```python
from build123d import *

# Parameters (mm, degrees)
SKETCH28_W          = 12.7
SKETCH28_H          = 12.7
BOSS_EXTRUDE5_DEPTH = 9.525
SKETCH29_W          = 12.7
SKETCH29_H          = 12.7
BOSS_EXTRUDE6_DEPTH = 9.525
SKETCH30_R          = 2.286
CUT_EXTRUDE7_DEPTH  = 270.036783662
SKETCH31_R          = 1.905
CUT_EXTRUDE8_DEPTH  = 12.7


with BuildPart() as part:
    # Sketch26 → Loft1 section 0
    with BuildSketch(Plane.XY):
        with BuildLine():
            Line((-6.35, 6.35), (6.35, 6.35))
            Line((6.35, 6.35), (6.35, -6.35))
            Line((6.35, -6.35), (-6.35, -6.35))
            Line((-6.35, -6.35), (-6.35, 6.35))
        make_face()
    # Sketch27 → Loft1 section 1
    with BuildSketch(Plane.XY.offset(238.245840754)):
        with BuildLine():
            Line((-49.2125, -88.9), (-61.9125, -88.9))
            Line((-61.9125, -88.9), (-61.9125, -76.2))
            Line((-61.9125, -76.2), (-49.2125, -76.2))
            Line((-49.2125, -76.2), (-49.2125, -88.9))
        make_face()
    loft()

    # Sketch28 → Boss-Extrude5 (add)
    with BuildSketch(Plane(origin=(0, 0, 0), x_dir=(-1, 0, 0), z_dir=(0, 0, -1))):
        Rectangle(SKETCH28_W, SKETCH28_H)
    extrude(amount=BOSS_EXTRUDE5_DEPTH)

    # Sketch29 → Boss-Extrude6 (add)
    with BuildSketch(Plane.XY.offset(238.245840754)):
        with Locations((-55.5625, -82.55)):
            Rectangle(SKETCH29_W, SKETCH29_H)
    extrude(amount=BOSS_EXTRUDE6_DEPTH)

    # Sketch30 → Cut-Extrude7 (cut, through all)
    with BuildSketch(Plane(origin=(-49.2125, 0, 0), x_dir=(0, 0, -1), z_dir=(1, 0, 0))):
        with Locations(Location((-243.008340754, -82.55, 0), (0, 0, 90))):
            Circle(SKETCH30_R)
    extrude(amount=-CUT_EXTRUDE7_DEPTH, mode=Mode.SUBTRACT)

    # Sketch31 → Cut-Extrude8 (cut)
    with BuildSketch(Plane(origin=(0, 0, -9.525), x_dir=(-1, 0, 0), z_dir=(0, 0, -1))):
        Circle(SKETCH31_R)
    extrude(amount=-CUT_EXTRUDE8_DEPTH, mode=Mode.SUBTRACT)


solid = part.part
```
Input: part model. Units: mm. Frame: model coordinates. A direction names the side the tool comes from. Coordinates: 2 decimals unless noted, no trailing zeros. Use a Markdown table: item, result. Add a question column.
1) Pin query (flat end, axial travel): P1, Ø3, axis at x = -55.5, z = 240.5, coming from the +Y side; P2, Ø1.1, axis at x = 0.5, y = 0, coming from the -Z side (3 decimals); P3, Ø3, axis at y = -79.5, z = 243, coming from the +X side. Return the tip coordinate at first contact, or that it passes through.
2) Draft query along Z for faces 1 (the flat face through (-61.912, -81, 245)), 2 (the flat face through (-56, -82, 247.771)), 3 (the cylindrical face through (-55.47, -80.37, 243.69)). Return one class per face: +Z half, -Z half, draft (parallel to the pull), parting line (faces both ways), or undercut.
3) Line query: L1, parallel to Y at x = 0, z = -6 (3 decimals); L2, parallel to X at y = -55, z = 176; L3, parallel to Y at x = -36.5, z = 137. Output: solid intervals per line, ascending. Write a range as from..to.
4) Set-up query: faces 4 (the flat face through (-6.35, 0, -5)), 5 (the flat face through (-56, -76.2, 243)), 6 (the flat face through (0, -6.35, -5)). Return all of +Z, -Z, +X, -X, +Y, -Y with unobstructed straight access to the full face (end or side cutting, diameter ignored); none if empty.
Answer below:
| question | item | result |
|---|---|---|
| 1 | P1 | y = -76.2 |
| 1 | P2 | z = 3.175 |
| 1 | P3 | x = -49.21 |
| 2 | face 1 | draft |
| 2 | face 2 | +Z half |
| 2 | face 3 | undercut |
| 3 | L1 | -6.35..-1.905, 1.905..6.35 |
| 3 | L2 | -47.4..-34.7 |
| 3 | L3 | -53.82..-41.12 |
| 4 | face 4 | -Z, -X, +Y, -Y |
| 4 | face 5 | +Z, +X, -X, +Y |
| 4 | face 6 | -Z, +X, -X, -Y |
